Job drawing, mm, ordinate dimensions from the low corner. One solid piece. A direction names the side the tool comes from. Give positions to 0.01 mm unless a question says otherwise; leave off trailing zeros. Write each loop counter-clockwise with the first axis right and the second up, starting at its lowest first coordinate (ties: lowest second). Pieces come first, ordered by that corner, then holes. Notation, with made-up numbers: M -19.5,66 L 35.5,66 A28 ccw 35.5,104 Z; hole C 27,65 d3. An arc over 180 degrees is marked long. Answer as CSV lines item,"result". Start each with the question number.
1) Pin check, flat tip, straight feed: pin 1 Ø12 at (y, z) = (19.5, 21.5) entering from +X. Stop position of the tip, or through.
2) Slice it at B-B, the plane x = 3.55. Give the cut face in (y, z).
3) Wall check: line 1 along Z through (x, y) = (1.4, 20.25); line 2 along Y through (x, z) = (2.35, 31.5). Give the ranges that are in metal, low to high. Write a range as from..to.
4) Tool access for the marked faces 4 and 5: list every direction of +Z, -Z, +X, -X, +Y, -Y with a clear straight run to the whole face (end or side of a thin tool).
5) Mould opens along Z. For the marked faces 1, 2 and 3 say: pulls with the +Z half, pulls with the -Z half, needs draft (parallel to the pull), parting line crosses it, or undercut.
6) Slice it at A-A, the plane z = 10. Give the cut face in (x, y).
7) Slice it at C-C, the plane y = 19. Give the cut face in (x, z), plus the area to 3 significant figures.
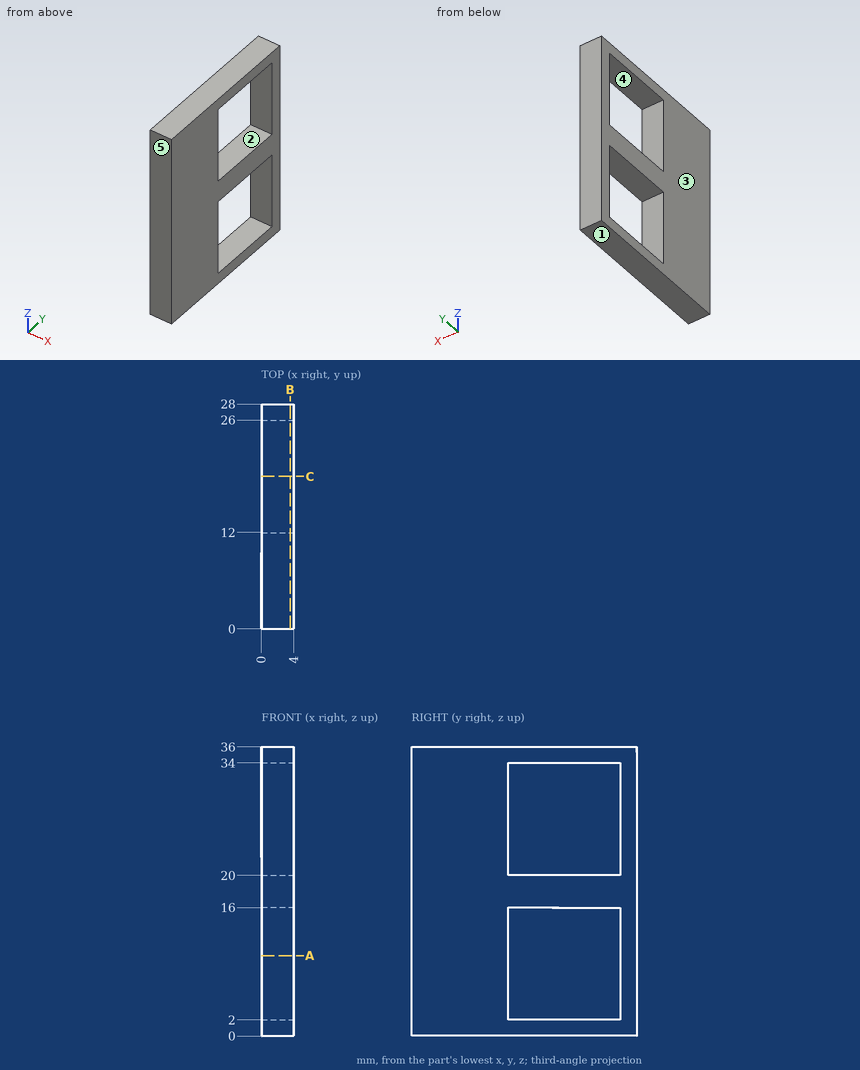
Found:
1,pin 1,"x = 4"
2,outline,"M 0,0 L 28,0 L 28,36 L 0,36 Z; hole M 12,2 L 26,2 L 26,16 L 12,16 Z; hole M 12,20 L 26,20 L 26,34 L 12,34 Z"
3,line 1,"0..2, 16..20, 34..36"
3,line 2,"0..12, 26..28"
4,face 4,"+X, -X"
4,face 5,"+Z, -Z, +X, -X, -Y"
5,face 1,"pulls with the -Z half"
5,face 2,"undercut"
5,face 3,"needs draft"
6,outline,"M 0,0 L 4,0 L 4,12 L 0,12 Z; M 0,26 L 4,26 L 4,28 L 0,28 Z"
7,outline,"M 0,0 L 4,0 L 4,2 L 0,2 Z; M 0,16 L 4,16 L 4,20 L 0,20 Z; M 0,34 L 4,34 L 4,36 L 0,36 Z"
7,area,"32.0 mm²"
